from build123d import *

# Parameters (mm, degrees)
SKETCH1_W           = 304.8
SKETCH1_H           = 381
BOSS_EXTRUDE1_DEPTH = 17.78
SKETCH2_W           = 88.9
SKETCH2_H           = 114.3
CUT_EXTRUDE1_DEPTH  = 12.7
SKETCH3_W           = 279.4
SKETCH3_H           = 355.6
CUT_EXTRUDE2_DEPTH  = 2.54
SKETCH4_R           = 1.27
CUT_EXTRUDE3_DEPTH  = 12.7


with BuildPart() as part:
    # Sketch1 → Boss-Extrude1 (new body)
    with BuildSketch(Plane.XY):
        with Locations((152.4, 190.5)):
            Rectangle(SKETCH1_W, SKETCH1_H)
    extrude(amount=BOSS_EXTRUDE1_DEPTH)

    # Sketch2 → Cut-Extrude1 (cut)
    with BuildSketch(Plane.XY.offset(17.78)):
        with Locations((57.15, 69.85)):
            Rectangle(SKETCH2_W, SKETCH2_H)
        with Locations((152.4, 311.15)):
            Rectangle(SKETCH2_W, SKETCH2_H)
        with Locations((57.15, 311.15)):
            Rectangle(SKETCH2_W, SKETCH2_H)
        with Locations((247.65, 311.15)):
            Rectangle(SKETCH2_W, SKETCH2_H)
        with Locations((57.15, 190.5)):
            Rectangle(SKETCH2_W, SKETCH2_H)
        with Locations((152.4, 190.5)):
            Rectangle(SKETCH2_W, SKETCH2_H)
        with Locations((247.65, 190.5)):
            Rectangle(SKETCH2_W, SKETCH2_H)
        with Locations((152.4, 69.85)):
            Rectangle(SKETCH2_W, SKETCH2_H)
        with Locations((247.65, 69.85)):
            Rectangle(SKETCH2_W, SKETCH2_H)
    extrude(amount=-CUT_EXTRUDE1_DEPTH, mode=Mode.SUBTRACT)

    # Sketch3 → Cut-Extrude2 (cut)
    with BuildSketch(Plane.XY.offset(17.78)):
        with Locations((152.4, 190.5)):
            Rectangle(SKETCH3_W, SKETCH3_H)
    extrude(amount=-CUT_EXTRUDE2_DEPTH, mode=Mode.SUBTRACT)

    # Sketch4 → Cut-Extrude3 (cut)
    with BuildSketch(Plane(origin=(0, 0, 0), x_dir=(-1, 0, 0), z_dir=(0, 0, -1))):
        with Locations((-6.35, 374.65)):
            Circle(SKETCH4_R)
        with Locations((-298.45, 374.65)):
            Circle(SKETCH4_R)
    extrude(amount=-CUT_EXTRUDE3_DEPTH, mode=Mode.SUBTRACT)


solid = part.part
Geometry: final body of the model. Coordinates: model frame, mm. A direction names the side the tool comes from. Give positions to 0.01 mm unless a question says otherwise; leave off trailing zeros. Order: outer loops, then holes, each group sorted by start corner. A loop starts at its lowest first (then second) coordinate and runs counter-clockwise, first axis right, second up. Notation, with made-up numbers: (29, 70) -> (73, 70) arc R30 ccw to (73, 92) -> close; hole circle Ø8 at (86, 71). An arc over 180 degrees is marked (long way). Answer as a JSON object with one key per item and string values.
Q1. Section B-B (y = 295.5). Output: boundary loops of the cut face in (x, z), plus the area to 3 significant figures.
Entries:
{"outline": "(0, 0) -> (304.8, 0) -> (304.8, 17.78) -> (292.1, 17.78) -> (292.1, 5.08) -> (203.2, 5.08) -> (203.2, 15.24) -> (196.85, 15.24) -> (196.85, 5.08) -> (107.95, 5.08) -> (107.95, 15.24) -> (101.6, 15.24) -> (101.6, 5.08) -> (12.7, 5.08) -> (12.7, 17.78) -> (0, 17.78) -> close", "area": "2,000 mm^2"}
Q2. Draft query along Y for faces 1 (the flat face through (107.95, 190, 10)), 2 (the flat face through (0, 188, 9)). Return one class per face: released by +Y, released by -Y, zero draft, split by the parting line, or undercut.
Entries:
{"face 1": "undercut", "face 2": "zero draft"}
Q3. Section A-A (x = 244). Output: boundary loops of the cut face in (y, z), plus the area to 3 significant figures.
Entries:
{"outline": "(0, 0) -> (381, 0) -> (381, 17.78) -> (368.3, 17.78) -> (368.3, 5.08) -> (254, 5.08) -> (254, 15.24) -> (247.65, 15.24) -> (247.65, 5.08) -> (133.35, 5.08) -> (133.35, 15.24) -> (127, 15.24) -> (127, 5.08) -> (12.7, 5.08) -> (12.7, 17.78) -> (0, 17.78) -> close", "area": "2,390 mm^2"}
Q4. Access query for faces 3 (the flat face through (247, 71, 5.08)), 4 (the flat face through (304.8, 188, 9)). Directions: +Z, -Z, +X, -X, +Y, -Y. A direction counts if a zero-diameter tool reaches every point of the face in a straight line with its end or side. Return the directions, or none.
Entries:
{"face 3": "+Z", "face 4": "+Z, -Z, +X, +Y, -Y"}
Q5. First-contact query: pin 1 (8 mm diameter, centred on y = 48.5, z = 11, fed in from -X); pin 2 (0.8 mm diameter, centred on x = 298, y = 375, fed in from -Z); pin 3 (10 mm diameter, centred on x = 120.5, y = 332.5, fed in from +Z); pin 4 (8 mm diameter, centred on x = 206, y = 231, fed in from +Z). Flat tips, straight axial feed; report the tip coordinate or a pass-through.
Entries:
{"pin 1": "stops at x = 0", "pin 2": "stops at z = 12.7", "pin 3": "stops at z = 5.08", "pin 4": "stops at z = 15.24"}
Q6. Material intervals for probe 1 along X at (y, z) = (303, 10.25); probe 2 along X at (y, z) = (374.65, 8.5); probe 3 along Y at (x, z) = (137.5, 5.5), sorted ascending.
Entries:
{"probe 1": "x = 0 to 12.7, 101.6 to 107.95, 196.85 to 203.2, 292.1 to 304.8", "probe 2": "x = 0 to 5.08, 7.62 to 297.18, 299.72 to 304.8", "probe 3": "y = 0 to 12.7, 127 to 133.35, 247.65 to 254, 368.3 to 381"}
